Read the model definition and answer for the solid it produces. Units are mm, in the model's axes. A direction names the side the tool comes from. Round coordinates to 2 decimals unless told otherwise and drop trailing zeros. Order: outer loops, then holes, each group sorted by start corner. A loop starts at its lowest first (then second) coordinate and runs counter-clockwise, first axis right, second up. Notation, with made-up numbers: (52, 40.25) -> (88, 40.25) arc R18 cw to (88, 69.25) -> close; hole circle Ø2 at (-26, 47.5). An arc over 180 degrees is marked (long way). Answer as a JSON object with one key per item and string values. Group by question number.
Item 1: Section B-B, the plane z = 0.25 is taken. Write down the section's boundary in (x, y) (3 decimals).
Item 2: The mould has two halves that part along Z. Classify faces 4 (the flat face through (-0.725, 5, -1)), 5 (the flat face through (0, 2, -4.295)), 6 (the flat face through (0, 3.52, 1)): pulls with the +Z half, pulls with the -Z half, needs draft (parallel to the pull), parting line crosses it, or undercut.
Item 3: For faces 1 (the flat face through (1.885, 2, 0)), 2 (the flat face through (0, 5, -1.675)), 3 (the flat face through (0.725, 5, -1)), determine the directions among +Z, -Z, +X, -X, +Y, -Y from which every point of the face is accessible in a straight line to the end or side of a thin tool.
Item 4: Consider probe 1 along Y at (x, z) = (-0.8, 3.25); probe 2 along X at (y, z) = (-4, 0) (3 decimals); probe 3 along Y at (x, z) = (-0.65, 0). Determine where each line is inside the solid, lowest interval first. Write a range as from..to.
Item 5: Section C-C, the plane x = 0 is taken. Write down the section's boundary in (y, z) (3 decimals).
Item 6: Section A-A, the plane y = -3.25 is taken. Write down the section's boundary in (x, z) (3 decimals), plus the area to 4 significant figures.
Item 7: Given P1, Ø1, axis at x = -0.5, y = 5, coming from the +Z side (3 decimals); P2, Ø2, axis at x = 0, z = -3.5, coming from the +Y side; P3, Ø1.2, axis at y = 5, z = -1, coming from the +X side (3 decimals), each flat-ended and moving along its own axis, determine where each tip first touches the part or whether it passes through.
Item 8: Section D-D, the plane y = 4.25 is taken. Write down the section's boundary in (x, z) (3 decimals), plus the area to 3 significant figures.
Autodesk Fusion 360 part; units mm, degrees
sketch "Sketch1" plane through (0, 0, 0) normal (0, 1, 0) x (1, 0, 0)
  line L0 (1.885, 4.295) -> (-1.885, 4.295)
  line L1 (-1.885, 4.295) -> (-1.885, -4.295)
  line L2 (-1.885, -4.295) -> (1.885, -4.295)
  line L3 (1.885, -4.295) -> (1.885, 4.295)
  line L4 (1.885, 4.295) -> (-1.885, -4.295) construction
  line L5 (-1.885, 4.295) -> (1.885, -4.295) construction
  dimension "d1" = 3.77
  dimension "d2" = 8.59
extrude "Extrude1" add sketch "Sketch1" along normal blind 3.77
sketch "Sketch2" plane through (0, 3.77, 0) normal (0, 1, 0) x (-1, 0, 0)
  line L0 (-1.885, 4.295) -> (-1.885, -4.295)
  line L1 (-1.885, -4.295) -> (1.885, -4.295)
  line L2 (1.885, -4.295) -> (1.885, 4.295)
  line L3 (1.885, 4.295) -> (-1.885, 4.295)
  line L4 (0.725, 1.675) -> (-0.725, 1.675)
  line L5 (-0.725, 1.675) -> (-0.725, -1.675)
  line L6 (-0.725, -1.675) -> (0.725, -1.675)
  line L7 (0.725, -1.675) -> (0.725, 1.675)
  line L8 (0.725, 1.675) -> (-0.725, -1.675) construction
  line L9 (-0.725, 1.675) -> (0.725, -1.675) construction
  dimension "d5" = 1.45
  dimension "d6" = 3.35
extrude "Extrude2" cut sketch "Sketch2" against normal blind 0.25 contours L4 L5 L6 L7
sketch "Sketch3" plane through (0, 3.52, 0) normal (0, 1, 0) x (-1, 0, 0)
  line L0 (0.725, -1.675) -> (0.725, 1.675)
  line L1 (0.725, 1.675) -> (-0.725, 1.675)
  line L2 (-0.725, 1.675) -> (-0.725, -1.675)
  line L3 (-0.725, -1.675) -> (0.725, -1.675)
  line L4 (0.725, -1.675) -> (-0.725, -1.675)
  line L5 (-0.725, -1.675) -> (-0.725, -0.225)
  line L6 (-0.725, -0.225) -> (0.725, -0.225)
  line L7 (0.725, -0.225) -> (0.725, -1.675)
  dimension "d9" = 1.45
  dimension "d10" = 1.45
extrude "Extrude3" add sketch "Sketch3" along normal blind 2.82 contours L0 L2 L3 L4 L5 L6 L7
sketch "Sketch4" plane through (0, 0, 0) normal (0, -1, 0) x (1, 0, 0)
  line L0 (1.885, -4.295) -> (1.885, 4.295)
  line L1 (1.885, 4.295) -> (-1.885, 4.295)
  line L2 (-1.885, 4.295) -> (-1.885, -4.295)
  line L3 (-1.885, -4.295) -> (1.885, -4.295)
  line L4 (0, -4.295) -> (0, 4.295) construction
  line L5 (1.885, 0) -> (-1.885, 0) construction
  line L6 (0.125, -0.125) -> (-0.125, -0.125)
  line L7 (-0.125, -0.125) -> (-0.125, 0.125)
  line L8 (-0.125, 0.125) -> (0.125, 0.125)
  line L9 (0.125, 0.125) -> (0.125, -0.125)
  line L10 (0.125, -0.125) -> (-0.125, 0.125) construction
  line L11 (-0.125, -0.125) -> (0.125, 0.125) construction
  line L12 (0.125, 2.7383) -> (-0.125, 2.7383)
  line L13 (-0.125, 2.7383) -> (-0.125, 2.9883)
  line L14 (-0.125, 2.9883) -> (0.125, 2.9883)
  line L15 (0.125, 2.9883) -> (0.125, 2.7383)
  line L16 (0.125, 2.7383) -> (-0.125, 2.9883) construction
  line L17 (-0.125, 2.7383) -> (0.125, 2.9883) construction
  line L18 (0.125, -2.9883) -> (0.125, -2.7383)
  line L19 (0.125, -2.7383) -> (-0.125, -2.7383)
  line L20 (-0.125, -2.7383) -> (-0.125, -2.9883)
  line L21 (-0.125, -2.9883) -> (0.125, -2.9883)
  point P0 (0, 2.8633)
  point P1 (0, -2.8633)
  dimension "d14" = 0.25
  dimension "d15" = 0.25
  dimension "d16" = 0.25
  dimension "d17" = 0.25
  dimension "d18" = 2.8633
extrude "Extrude4" add sketch "Sketch4" along normal blind 4.91 contours L6 L7 L8 L9 | L12 L13 L14 L15 | L18 L19 L20 L21
fillet "Fillet1" radius 0.25 4 edges at (1.885, 3.77, 0) (0, 3.77, 4.295) (0, 3.77, -4.295) (-1.885, 3.77, 0)
fillet "Fillet2" radius 0.25 4 edges at (0.725, 6.34, -0.95) (0, 6.34, -1.675) (-0.725, 6.34, -0.95) (0, 6.34, -0.225)
Values found:
{
 "1": {"outline": "(-1.885, 0) -> (1.885, 0) -> (1.885, 3.52) arc R0.25 ccw to (1.635, 3.77) -> (0.725, 3.77) -> (0.725, 3.52) -> (-0.725, 3.52) -> (-0.725, 3.77) -> (-1.635, 3.77) arc R0.25 ccw to (-1.885, 3.52) -> close"},
 "2": {"face 4": "needs draft", "face 5": "pulls with the -Z half", "face 6": "undercut"},
 "3": {"face 1": "+Z, -Z, +X, +Y, -Y", "face 2": "-Z, +X, -X, +Y", "face 3": "+Z, -Z, +X, +Y"},
 "4": {"probe 1": "0..3.77", "probe 2": "-0.125..0.125", "probe 3": "0..3.52"},
 "5": {"outline": "(-4.91, -2.988) -> (0, -2.988) -> (0, -4.295) -> (3.52, -4.295) arc R0.25 ccw to (3.77, -4.045) -> (3.77, -1.675) -> (6.09, -1.675) arc R0.25 ccw to (6.34, -1.425) -> (6.34, -0.475) arc R0.25 ccw to (6.09, -0.225) -> (3.52, -0.225) -> (3.52, 1.675) -> (3.77, 1.675) -> (3.77, 4.045) arc R0.25 ccw to (3.52, 4.295) -> (0, 4.295) -> (0, 2.988) -> (-4.91, 2.988) -> (-4.91, 2.738) -> (0, 2.738) -> (0, 0.125) -> (-4.91, 0.125) -> (-4.91, -0.125) -> (0, -0.125) -> (0, -2.738) -> (-4.91, -2.738) -> close"},
 "6": {"outline": "(-0.125, -2.988) -> (0.125, -2.988) -> (0.125, -2.738) -> (-0.125, -2.738) -> close; (-0.125, -0.125) -> (0.125, -0.125) -> (0.125, 0.125) -> (-0.125, 0.125) -> close; (-0.125, 2.738) -> (0.125, 2.738) -> (0.125, 2.988) -> (-0.125, 2.988) -> close", "area": "0.1875 mm2"},
 "7": {"P1": "z = -0.225", "P2": "y = 3.77", "P3": "x = 0.725"},
 "8": {"outline": "(-0.725, -1.675) -> (0.725, -1.675) -> (0.725, -0.225) -> (-0.725, -0.225) -> close", "area": "2.10 mm2"}
}
